Work out the finished part from the listing and answer in its coordinate system (mm). A direction names the side the tool comes from. Give positions to 0.01 mm unless a question says otherwise; leave off trailing zeros. Write each question's results on one line, items separated by ' | '.
from build123d import *

# Parameters (mm, degrees)
SKETCH1_R           = 60
BOSS_EXTRUDE1_DEPTH = 10
SKETCH2_R           = 90
BOSS_EXTRUDE2_DEPTH = 15
SKETCH3_R           = 45
BOSS_EXTRUDE3_DEPTH = 30
FILLET1_R           = 10
FILLET2_R           = 30


with BuildPart() as part:
    # Sketch1 → Boss-Extrude1 (new body)
    with BuildSketch(Plane(origin=(0, 0, 0), x_dir=(1, 0, 0), z_dir=(0, 1, 0))):
        with Locations(Location((0, 0, 0), (0, 0, 270))):
            Circle(SKETCH1_R)
    extrude(amount=BOSS_EXTRUDE1_DEPTH)

    # Sketch2 → Boss-Extrude2 (add)
    with BuildSketch(Plane(origin=(0, 10, 0), x_dir=(1, 0, 0), z_dir=(0, 1, 0))):
        with Locations(Location((0, 0, 0), (0, 0, 270))):
            Circle(SKETCH2_R)
    extrude(amount=BOSS_EXTRUDE2_DEPTH)

    # Sketch3 → Boss-Extrude3 (add)
    with BuildSketch(Plane(origin=(0, 25, 0), x_dir=(1, 0, 0), z_dir=(0, 1, 0))):
        with Locations(Location((0, 0, 0), (0, 0, 270))):
            Circle(SKETCH3_R)
    extrude(amount=BOSS_EXTRUDE3_DEPTH)

    # Fillet1
    fillet1_edges = [part.edges().sort_by_distance(p)[0] for p in [
        (0, 25, -90),
    ]]
    fillet(fillet1_edges, radius=FILLET1_R)

    # Fillet2
    fillet2_edges = [part.edges().sort_by_distance(p)[0] for p in [
        (0, 55, -45),
    ]]
    fillet(fillet2_edges, radius=FILLET2_R - 0.0001)  # a hair under: the kernel refuses the full size


solid = part.part
1. Given P1, Ø6, axis at x = 8, y = 46, coming from the +Z side; P2, Ø1.5, axis at y = 44.5, z = 3.5, coming from the -X side; P3, Ø1.5, axis at x = -18.5, z = 43.5, coming from the +Y side, each flat-ended and moving along its own axis, determine where each tip first touches the part or whether it passes through.
Answer list:
P1: z = 38.25 | P2: x = -38.26 | P3: y = 25
2. Straight lines are drawn through the part: line 1 (Y direction, x = 51, z = -36.5); line 2 (Y direction, x = -28, z = 43); line 3 (X direction, y = 6, z = -49). For each, find the intervals that lie inside material, in ascending order. Write a range as [from, to].
Answer list:
line 1: [10, 25] | line 2: [0, 25] | line 3: [-34.63, 34.63]
3. Determine the mould class of faces 1 (the face through (0, 55, 0)), 2 (the face through (1, 0, -1)), 3 (the face through (2.64, 4.93, -59.94)) for opening direction Y: +Y half, -Y half, draft (parallel to the pull), parting line (faces both ways), or undercut.
Answer list:
face 1: +Y half | face 2: -Y half | face 3: draft
4. A tool of negligible diameter and unlimited length cuts with its end or side. For faces 4 (the face through (-34, 25, 34)), 5 (the face through (-19, 10, 59)), 6 (the face through (-34.471, 12.465, 83.137)), from which of +Z, -Z, +X, -X, +Y, -Y can it reach the whole face along a straight path? Write none if from no direction.
Answer list:
face 4: +Y | face 5: -Y | face 6: +Y, -Y
